from build123d import *

# Parameters (mm, degrees)
SKETCH2_R                = 90
BOSS_EXTRUDE1_DEPTH      = 0.75
CUT_EXTRUDE2_DEPTH       = 0.75
CUT_EXTRUDE6_START       = -1.75
CUT_EXTRUDE6_DEPTH       = 2.5
CUT_EXTRUDE7_DEPTH       = 0.75
FILLET1_R                = 4
CIRPATTERN1_COUNT        = 4
CIRPATTERN2_COUNT        = 4
FILLET1_OF_CIRPATTERN2_R = 4
SKETCH9_R                = 3.5
CUT_EXTRUDE8_DEPTH       = 0.75
CIRPATTERN3_COUNT        = 4


with BuildPart() as part:
    # Sketch2 → Boss-Extrude1 (new body)
    with BuildSketch(Plane(origin=(0, 0, 0), x_dir=(1, 0, 0), z_dir=(0, 1, 0))):
        Circle(SKETCH2_R)
        with BuildLine():
            ThreePointArc((21.169734538, -7.621833087), (22.857266397, -9.097867547), (23.485571585, -11.25))
            ThreePointArc((23.485571585, -11.25), (21.32947872, -14.799648783), (17.185568345, -14.522611358))
            ThreePointArc((17.185568345, -14.522611358), (0, -22.5), (-17.185568345, -14.522611358))
            ThreePointArc((-17.185568345, -14.522611358), (-22.9496732, -13.25), (-21.169734538, -7.621833087))
            ThreePointArc((-21.169734538, -7.621833087), (-19.485571585, 11.25), (-3.984166192, 22.144444444))
            ThreePointArc((-3.984166192, 22.144444444), (-0.177953971, 26.496039587), (4, 22.5))
            ThreePointArc((4, 22.5), (3.996039587, 22.322046029), (3.984166192, 22.144444444))
            ThreePointArc((3.984166192, 22.144444444), (17.261137554, 14.432710429), (22.5, 0))
            ThreePointArc((22.5, 0), (22.164938835, -3.8685251), (21.169734538, -7.621833087))
        make_face(mode=Mode.SUBTRACT)
    extrude(amount=BOSS_EXTRUDE1_DEPTH)

    # Sketch4 → Cut-Extrude2 (cut)
    with BuildSketch(Plane(origin=(0, 0.75, 0), x_dir=(1, 0, 0), z_dir=(0, 1, 0))):
        with BuildLine():
            Line((-18.75, 34.75), (18.75, 34.75))
            ThreePointArc((18.75, 34.75), (28.059393859, 42.356541264), (22.4609375, 52.995224003))
            ThreePointArc((22.4609375, 52.995224003), (0, 57.563605035), (-22.4609375, 52.995224003))
            ThreePointArc((-22.4609375, 52.995224003), (-28.059393859, 42.356541264), (-18.75, 34.75))
        make_face()
    cut_extrude2 = extrude(amount=-CUT_EXTRUDE2_DEPTH, mode=Mode.SUBTRACT)

    # Sketch7 → Cut-Extrude6 (cut)
    with BuildSketch(Plane(origin=(0, 0.75, 0), x_dir=(1, 0, 0), z_dir=(0, 1, 0)).offset(CUT_EXTRUDE6_START)):
        with BuildLine():
            Line((50.187203194, 48.078005736), (65, 62.24949799))
            ThreePointArc((65, 62.24949799), (62.546689472, 64.714076027), (60, 67.082039325))
            Line((60, 67.082039325), (46.326130039, 51.8086834))
            ThreePointArc((46.326130039, 51.8086834), (31.405257095, 61.999676022), (14.361623616, 67.99995417))
            ThreePointArc((14.361623616, 67.99995417), (12.287770938, 66.649348724), (13.638376384, 64.575496046))
            ThreePointArc((13.638376384, 64.575496046), (35.62942383, 55.556675185), (52.99956323, 39.332509421))
            ThreePointArc((52.99956323, 39.332509421), (55.447762126, 38.970125419), (55.810146129, 41.418324315))
            ThreePointArc((55.810146129, 41.418324315), (53.103176506, 44.836398662), (50.187203194, 48.078005736))
        make_face()
    cut_extrude6 = extrude(amount=CUT_EXTRUDE6_DEPTH, mode=Mode.SUBTRACT)

    # Sketch8 → Cut-Extrude7 (cut)
    with BuildSketch(Plane(origin=(0, 0.75, 0), x_dir=(1, 0, 0), z_dir=(0, 1, 0))):
        Polygon((-25.925493975, 21.336832502), (-31.229304965, 27.056062257), (-26.683250545, 31.271912018), (-21.379439555, 25.552682263), align=None)
    cut_extrude7 = extrude(amount=-CUT_EXTRUDE7_DEPTH, mode=Mode.SUBTRACT)

    # Fillet1
    fillet1_edges = [part.edges().sort_by_distance(p)[0] for p in [
        (50.187203194, 0.375, -48.078005736),
        (46.326130039, 0.375, -51.8086834),
    ]]
    fillet(fillet1_edges, radius=FILLET1_R)

    # CirPattern1: Cut-Extrude2, Cut-Extrude7 ×4 about axis
    cirpattern1_axis = Axis((0, 0, 0), (0, 1, 0))
    for i in range(1, CIRPATTERN1_COUNT):
        add(cut_extrude2.rotate(cirpattern1_axis, i * 360 / CIRPATTERN1_COUNT), mode=Mode.SUBTRACT)
        add(cut_extrude7.rotate(cirpattern1_axis, i * 360 / CIRPATTERN1_COUNT), mode=Mode.SUBTRACT)

    # CirPattern2: Cut-Extrude6 ×4 about axis
    cirpattern2_axis = Axis((0, 0, 0), (0, 1, 0))
    for i in range(1, CIRPATTERN2_COUNT):
        add(cut_extrude6.rotate(cirpattern2_axis, i * 360 / CIRPATTERN2_COUNT), mode=Mode.SUBTRACT)

    # Fillet1 of CirPattern2
    fillet1_of_cirpattern2_edges = [part.edges().sort_by_distance(p)[0] for p in [
        (-48.078005736, 0.375, -50.187203194),
        (-51.8086834, 0.375, -46.326130039),
        (-50.187203194, 0.375, 48.078005736),
        (-46.326130039, 0.375, 51.8086834),
        (48.078005736, 0.375, 50.187203194),
        (51.8086834, 0.375, 46.326130039),
    ]]
    fillet(fillet1_of_cirpattern2_edges, radius=FILLET1_OF_CIRPATTERN2_R)

    # Sketch9 → Cut-Extrude8 (cut)
    with BuildSketch(Plane(origin=(0, 0.75, 0), x_dir=(1, 0, 0), z_dir=(0, 1, 0))):
        with Locations((-36.860788245, 38.982108588)):
            Circle(SKETCH9_R)
    cut_extrude8 = extrude(amount=-CUT_EXTRUDE8_DEPTH, mode=Mode.SUBTRACT)

    # CirPattern3: Cut-Extrude8 ×4 about axis
    cirpattern3_axis = Axis((0, 0, 0), (0, 1, 0))
    for i in range(1, CIRPATTERN3_COUNT):
        add(cut_extrude8.rotate(cirpattern3_axis, i * 360 / CIRPATTERN3_COUNT), mode=Mode.SUBTRACT)


solid = part.part
Check sheet for the modelled part. Datum: model origin and axes. Units: mm. Round coordinates to 2 decimals unless told otherwise and drop trailing zeros. Write each loop counter-clockwise with the first axis right and the second up, starting at its lowest first coordinate (ties: lowest second). Pieces come first, ordered by that corner, then holes. Notation, with made-up numbers: (89, 77) - (104, 77) arc R32 ccw to (104, 116) - close; hole circle Ø5 at (83, -19.75). An arc over 180 degrees is marked (long way). Return JSON: item names as keys, results as strings.
Q1. Cross-section at C-C (z = 79.5). Record the boundary of the cut face in (x, y).
Returned:
{"outline": "(-42.19, 0) - (42.19, 0) - (42.19, 0.75) - (-42.19, 0.75) - close"}
Q2. Cross-section at A-A (x = 0). Record the boundary of the cut face in (y, z), then the cut area to 3 significant figures.
Returned:
{"outline": "(0, -90) - (0.75, -90) - (0.75, -57.56) - (0, -57.56) - close; (0, -34.75) - (0.75, -34.75) - (0.75, -26.5) - (0, -26.5) - close; (0, 22.5) - (0.75, 22.5) - (0.75, 34.75) - (0, 34.75) - close; (0, 57.56) - (0.75, 57.56) - (0.75, 90) - (0, 90) - close", "area": "64.0 mm²"}
Q3. Scan lines: L1, parallel to X at y = 0.1, z = 42; L2, parallel to X at y = 0.5, z = -7; L3, parallel to X at y = 0.25, z = 11.25. Record each from-to range of solid material in increasing order. Write a range as from..to.
Returned:
{"L1": "x = -79.6..-55.37, -50.91..-27.98, 27.98..35.09, 38.63..50.91, 55.37..79.6", "L2": "x = -89.73..-57.14, -34.75..-21.38, 21.38..34.75, 57.14..89.73", "L3": "x = -89.29..-56.45, -34.75..-23.49, 23.49..34.75, 56.45..89.29"}
Q4. Cross-section at B-B (y = 0.6). Give the number of separate pieces and of enclosed holes in the cut face, then the cut area to 3 significant figures.
Returned:
{"separate pieces": "1", "enclosed holes": "13", "area": "17,800 mm²"}
Q5. Cross-section at D-D (x = -77.5). Record the boundary of the cut face in (y, z), then the cut area to 3 significant figures.
Returned:
{"outline": "(0, -45.76) - (0.75, -45.76) - (0.75, 45.76) - (0, 45.76) - close", "area": "68.6 mm²"}
Q6. Draft check along Z on faces 1 (the flat face through (19, 0.75, 19)), 2 (the cylindrical face through (-0.6, 0.4, -90)), 3 (the flat face through (28.452, 0.38, -24.068)). Enter one of: released by +Z, released by -Z, zero draft, split by the parting line, or undercut.
Returned:
{"face 1": "zero draft", "face 2": "released by -Z", "face 3": "undercut"}
